The listing builds one solid part. Answer for the finished solid, in the listing's coordinates (mm). Face numbers are marked on the shaded views. A direction names the side the tool comes from. Round coordinates to 2 decimals unless told otherwise and drop trailing zeros. Order: outer loops, then holes, each group sorted by start corner. A loop starts at its lowest first (then second) coordinate and runs counter-clockwise, first axis right, second up. Notation, with made-up numbers: M 32.5,12 L 75.5,12 A18 cw 75.5,47 Z; hole C 0,61.5 d11. An arc over 180 degrees is marked long. Put each result on its own line as item: value. Start each with the question number.
1. The part is cut by section C-C (x = 7.5). Give the vertices of the cut face in (y, z), then the cut area to 4 significant figures.
2. The part is cut by section A-A (z = 13.5). Give the vertices of the cut face in (x, y).
3. Each of these flat-tipped pins is pushed along its axis until it touches: pin 1 Ø1.9 at (y, z) = (6.5, 4) entering from +X (3 decimals); pin 2 Ø5 at (y, z) = (-0.5, 2.5) entering from -X (3 decimals); pin 3 Ø7.5 at (x, y) = (-3.5, -1.5) entering from +Z. Where does it stop, or does it pass through?
4. The part is cut by section B-B (y = 5.5). Give the vertices of the cut face in (x, z) (3 decimals).
5. Which of the six approach directions +Z, -Z, +X, -X, +Y, -Y give full straight-line access (tool end or side, diameter ignored) to the marked faces 4, 5 and 6?
6. Consider line 1 (Y direction, x = 10, z = 15); line 2 (Z direction, x = -4, y = 10.5). Determine where each line is inside the solid, lowest interval first.
7. The mould has two halves that part along Y. Classify the marked faces 1, 2 and 3: +Y half, -Y half, draft (parallel to the pull), parting line (faces both ways), or undercut.
8. The part is cut by section D-D (y = 14). Give the vertices of the cut face in (x, z) (3 decimals), then the cut area to 3 significant figures.
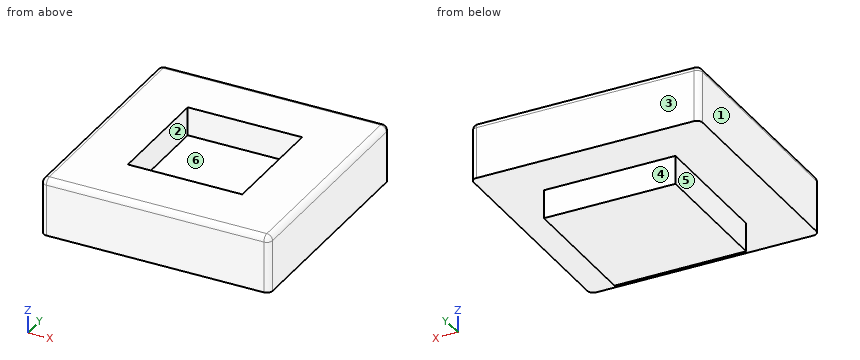
from build123d import *

# Parameters (mm, degrees)
F0_W     = 29.21
F0_H     = 29.972
F1_DEPTH = 6.35
F2_W     = 50.8
F2_H     = 50.8
F3_DEPTH = 12.7
F4_W     = 25.4
F4_H     = 25.4
F5_DEPTH = 6.35
F6_R     = 1.27


with BuildPart() as f1:
    # F0 (on Top) → F1 (new body)
    with BuildSketch(Plane.XY):
        Rectangle(F0_W, F0_H)
    extrude(amount=F1_DEPTH)

    # F2 (on face) → F3 (join)
    with BuildSketch(Plane.XY.offset(6.35)):
        Rectangle(F2_W, F2_H)
    extrude(amount=F3_DEPTH)

    # F4 (on face) → F5 (cut)
    with BuildSketch(Plane.XY.offset(19.05)):
        Rectangle(F4_W, F4_H)
    extrude(amount=-F5_DEPTH, mode=Mode.SUBTRACT)

    # F6
    f6_edges = [f1.edges().sort_by_distance(p)[0] for p in [
        (-25.4, -25.4, 12.7),
        (25.4, -25.4, 12.7),
        (25.4, 25.4, 12.7),
        (-25.4, 25.4, 12.7),
        (0, -25.4, 19.05),
        (-25.4, 0, 19.05),
        (0, 25.4, 19.05),
        (25.4, 0, 19.05),
    ]]
    fillet(f6_edges, radius=F6_R)


solid = f1.part
Resolved:
1. outline: M -25.4,6.35 L -14.99,6.35 L -14.99,0 L 14.99,0 L 14.99,6.35 L 25.4,6.35 L 25.4,17.78 A1.27 ccw 24.13,19.05 L 12.7,19.05 L 12.7,12.7 L -12.7,12.7 L -12.7,19.05 L -24.13,19.05 A1.27 ccw -25.4,17.78 Z
1. area: 673.5 mm2
2. outline: M -25.4,-24.13 A1.27 ccw -24.13,-25.4 L 24.13,-25.4 A1.27 ccw 25.4,-24.13 L 25.4,24.13 A1.27 ccw 24.13,25.4 L -24.13,25.4 A1.27 ccw -25.4,24.13 Z; hole M -12.7,-12.7 L 12.7,-12.7 L 12.7,12.7 L -12.7,12.7 Z
3. pin 1: x = 14.605
3. pin 2: x = -14.605
3. pin 3: z = 12.7
4. outline: M -25.4,6.35 L -14.605,6.35 L -14.605,0 L 14.605,0 L 14.605,6.35 L 25.4,6.35 L 25.4,17.78 A1.27 ccw 24.13,19.05 L 12.7,19.05 L 12.7,12.7 L -12.7,12.7 L -12.7,19.05 L -24.13,19.05 A1.27 ccw -25.4,17.78 Z
5. face 4: -Z, +X, -X, +Y
5. face 5: -Z, -X, +Y, -Y
5. face 6: +Z
6. line 1: -25.4 to -12.7, 12.7 to 25.4
6. line 2: 0 to 12.7
7. face 1: draft
7. face 2: undercut
7. face 3: +Y half
8. outline: M -25.4,6.35 L -14.605,6.35 L -14.605,0 L 14.605,0 L 14.605,6.35 L 25.4,6.35 L 25.4,17.78 A1.27 ccw 24.13,19.05 L -24.13,19.05 A1.27 ccw -25.4,17.78 Z
8. area: 830 mm2
